Solid Edge part; units mm, degrees
sketch "Sketch1" plane through (0, 0, 0) normal (0, -1, 0) x (1, 0, 0)
  line L0 (-109.896, -8.7564) -> (-39.896, 10)
  line L1 (-39.896, 10) -> (30.104, 10)
  arc A0 (30.104, 10) -> (30.104, -10) centre (30.104, 0) cw
  line L2 (30.104, -10) -> (-39.896, -10)
  line L3 (-39.896, -10) -> (-39.896, -18.7564)
  line L4 (-39.896, -18.7564) -> (-109.896, -18.7564)
  line L5 (-109.896, -18.7564) -> (-109.896, -8.7564)
  circle A1 centre (30.104, 0) radius 5
  circle A2 centre (0, 0) radius 5
  dimension "D1" = 39.896
  dimension "D2" = 39.896
  dimension "D3" = 109.896
  dimension "D4" = 39.896
extrude "Protrusion1" add sketch "Sketch1" along normal mid plane 4
sketch "Sketch2" plane through (-34.896, 0, -4.3782) normal (0, -1, 0) x (1, 0, 0)
  line L0 (-5, 14.3782) -> (-5, -20.6218)
  line L1 (-5, -20.6218) -> (-75, -14.7884)
  line L2 (-75, -4.3782) -> (-75, -14.7884)
  line L3 (-75, -4.3782) -> (-5, 14.3782)
  dimension "D1" = 5
  dimension "D2" = 5
extrude "Protrusion2" add sketch "Sketch2" along normal mid plane 15
sketch "Sketch3" plane through (-74.896, -7.5, -22.0833) normal (0.9965458, 0, -0.0830455) x (0, 1, 0)
  line L0 (7.5, 4) -> (3.5, 0)
  line L1 (3.5, 0) -> (11.5, 0)
  line L2 (7.5, 4) -> (11.5, 0)
  dimension "D1" = 7.5
extrude "Cutout1" cut sketch "Sketch3" along normal through all and the other way through all
sketch "Sketch4" plane through (-74.896, -7.5, -7.5) normal (0, -1, 0) x (0, 0, -1)
  line L0 (2.5, 128.4627) -> (2.5, -36.5848)
  line L1 (2.5, -36.5848) -> (-39.0806, -36.5848)
  line L2 (-39.0806, 128.4627) -> (-39.0806, -36.5848)
  line L3 (2.5, 128.4627) -> (-39.0806, 128.4627)
extrude "Cutout2" cut sketch "Sketch4" against normal up to next
sketch "Sketch5" plane through (-109.896, 0, -14.5833) normal (-1, 0, 0) x (0, 0, 1)
  line L0 (4.5833, -2) -> (4.5833, 2)
  line L1 (1.5833, 2) -> (4.5833, 2)
  line L2 (1.5833, 2) -> (1.5833, -2)
  line L3 (1.5833, -2) -> (4.5833, -2)
  dimension "D1" = 1.5833
  dimension "D2" = 1.5833
extrude "Cutout3" cut sketch "Sketch5" against normal up to next
sketch "Sketch6" plane through (-74.896, 0, -17) normal (0, 0, 1) x (1, 0, 0)
  circle A0 centre (30, 0) radius 4
  circle A1 centre (-5, 0) radius 4
extrude "VaciadoExtruido_6" cut sketch "Sketch6" against normal up to next
hole "Agujero_7" at (-79.896, 0, -17) direction (0, 0, 1) diameter 2.459 depth 7 tip angle 90 countersink diameter 6.94 countersink angle 90 thread major 3 thread length 5
hole "Hole1" at (-44.896, 0, -17) direction (0, 0, 1) diameter 2.459 depth 7 tip angle 90 countersink diameter 6.94 countersink angle 90 thread major 3 thread length 5
properties part number "1976-1500-006" material "Aluminio, 7075-T6"
Here's how the part is built. I have some questions about the finished solid (model axes, mm). A direction names the side the tool comes from. Round coordinates to 2 decimals unless told otherwise and drop trailing zeros. Loops run counter-clockwise (first coordinate to the right, second up) from the corner with the lowest first, then second, coordinate; pieces in that order, holes last. Notation, with made-up numbers: (54, 1.5) -> (75, 1.5) arc R30 cw to (75, 28.5) -> close; hole circle Ø1 at (8, 46.25). An arc over 180 degrees is marked (long way). Answer as CSV lines item,"result". Start each with the question number.
1. I'm going to push flat-ended pins straight in: P1, Ø3, axis at x = -44.896, y = 0, coming from the +Z side; P2, Ø9, axis at x = -80, y = -1.5, coming from the -Z side; P3, Ø1, axis at x = -62, y = -0.5, coming from the -Z side; P4, Ø9, axis at x = -44.896, y = 0, coming from the +Z side. Where does each tip first touch, or does it pass through?
2. Imagine slicing it at A-A on x = -97.5. Write out the boundary of the cut face in (y, z), plus the area to 3 significant figures.
3. If we mould it in two halves opening along Y, with no side actions, what happens to faces 6 (the face through (-95.11, -1.97, -18.36)), 7 (the face through (-74.406, -5.726, -22.124)), 8 (the face through (-74, 7.5, -16))? For each: pulls with the +Y half, pulls with the -Y half, needs draft (parallel to the pull), parting line crosses it, or undercut.
4. Imagine slicing it at B-B on y = 5. Write out the boundary of the cut face in (x, z).
5. For faces 1 (the face through (-74, -7.5, -16)), 2 (the face through (-83, 2, -17)), 3 (the face through (-109.896, 0, -15)), 4 (the face through (-75, 2, -12)), 5 (the face through (-62.47, -1.97, -21.08)), which set-ups out of +Z, -Z, +X, -X, +Y, -Y let a thin tool reach every point of the face, with its end or its side?
6. I need wall thicknesses on probe 1 along X at (y, z) = (0, -14.1); probe 2 along Y at (x, z) = (-75.5, -12); probe 3 along X at (y, z) = (-0.5, -14.25). Which ranges of each line are inside material? Lowest first, please. Write a range as from..to.
Solution:
1,P1,"z = -13"
1,P2,"z = -21.97"
1,P3,"z = -20.15"
1,P4,"z = -10"
2,outline,"(-7.5, -20.2) -> (-4, -20.2) -> (0, -16.19) -> (4, -20.2) -> (7.5, -20.2) -> (7.5, -10) -> (2, -10) -> (2, -13) -> (-2, -13) -> (-2, -10) -> (-7.5, -10) -> close"
2,area,"125 mm²"
3,face 6,"undercut"
3,face 7,"needs draft"
3,face 8,"pulls with the +Y half"
4,outline,"(-109.9, -19.17) -> (-39.9, -25) -> (-39.9, -10) -> (-109.9, -10) -> close"
5,face 1,"+Z, -Z, +X, -X, -Y"
5,face 2,"-Z"
5,face 3,"+Z, -Z, -X, +Y, -Y"
5,face 4,"+Z, +X, -X"
5,face 5,"-Z, -X"
6,probe 1,"-109.9..-81.13, -78.67..-46.13, -43.67..-39.9"
6,probe 2,"-7.5..-2, 2..7.5"
6,probe 3,"-109.9..-81.02, -78.77..-46.02, -43.77..-39.9"
